from build123d import *

# Parameters (mm, degrees)
SKETCH_1_W          = 95
SKETCH_1_H          = 38.85
EXTRUDE_1_DEPTH     = 1
SKETCH_2_W          = 11.4
SKETCH_2_H          = 15.06
SKETCH_2_W_2        = 24.986714953
SKETCH_2_H_2        = 25.25
SKETCH_2_W_3        = 12.976860002
SKETCH_2_H_3        = 16.4084
CUT_EXTRUDE_1_DEPTH = 10


with BuildPart() as part:
    # Эскиз1 → Бобышка-Вытянуть1 (new body)
    with BuildSketch(Plane(origin=(0.5, 0, 0), x_dir=(0, -1, 0), z_dir=(-1, 0, 0))):
        with Locations((-53.35, 22.825)):
            Rectangle(SKETCH_1_W, SKETCH_1_H)
    extrude(amount=-EXTRUDE_1_DEPTH)

    # Эскиз2 → Вырез-Вытянуть1 (cut)
    with BuildSketch(Plane.ZY.offset(-0.5)):
        with Locations((10.95, 17.108135831)):
            Rectangle(SKETCH_2_W, SKETCH_2_H)
        with Locations((15.906642524, 76.225)):
            Rectangle(SKETCH_2_W_2, SKETCH_2_H_2)
        with Locations((11.944169999, 33.813361354)):
            Rectangle(SKETCH_2_W_3, SKETCH_2_H_3)
    extrude(amount=-CUT_EXTRUDE_1_DEPTH, mode=Mode.SUBTRACT)


solid = part.part
Geometry: final body of the model. Coordinates: model frame, mm. Give positions to 0.01 mm unless a question says otherwise; leave off trailing zeros. Write each loop counter-clockwise with the first axis right and the second up, starting at its lowest first coordinate (ties: lowest second). Pieces come first, ordered by that corner, then holes.
(1) Cut plane C-C, the plane x = 1.1. Return loops of the section in (y, z), then the cut area to 3 significant figures.
(2) Cut plane A-A, the plane y = 40.5. Return loops of the section in (x, z).
(3) Ray query, line 1 (Y direction, x = 0.95, z = 14.5); line 2 (Y direction, x = 0.7, z = 21); line 3 (Z direction, x = 1.15, y = 16). Return the intervals inside material, ascending.
(4) Cut plane D-D, the plane y = 21. Return loops of the section in (x, z), then the cut area to 4 significant figures.
(5) Cut plane B-B, the plane z = 17.5. Return loops of the section in (x, y).
Values follow:
1. outline: (5.85, 3.4) - (100.85, 3.4) - (100.85, 42.25) - (5.85, 42.25) - close; hole (9.58, 5.25) - (24.64, 5.25) - (24.64, 16.65) - (9.58, 16.65) - close; hole (25.61, 5.46) - (42.02, 5.46) - (42.02, 18.43) - (25.61, 18.43) - close; hole (63.6, 3.41) - (88.85, 3.41) - (88.85, 28.4) - (63.6, 28.4) - close
1. area: 2,680 mm2
2. outline: (0.5, 3.4) - (1.5, 3.4) - (1.5, 5.46) - (0.5, 5.46) - close; (0.5, 18.43) - (1.5, 18.43) - (1.5, 42.25) - (0.5, 42.25) - close
3. line 1: y = 5.85 to 9.58, 24.64 to 25.61, 42.02 to 63.6, 88.85 to 100.85
3. line 2: y = 5.85 to 63.6, 88.85 to 100.85
3. line 3: z = 3.4 to 5.25, 16.65 to 42.25
4. outline: (0.5, 3.4) - (1.5, 3.4) - (1.5, 5.25) - (0.5, 5.25) - close; (0.5, 16.65) - (1.5, 16.65) - (1.5, 42.25) - (0.5, 42.25) - close
4. area: 27.45 mm2
5. outline: (0.5, 5.85) - (1.5, 5.85) - (1.5, 25.61) - (0.5, 25.61) - close; (0.5, 42.02) - (1.5, 42.02) - (1.5, 63.6) - (0.5, 63.6) - close; (0.5, 88.85) - (1.5, 88.85) - (1.5, 100.85) - (0.5, 100.85) - close
